The model under review builds one solid part; all positions refer to its coordinate system, in mm. A direction names the side the tool comes from. Round coordinates to 2 decimals unless told otherwise and drop trailing zeros. Order: outer loops, then holes, each group sorted by start corner. A loop starts at its lowest first (then second) coordinate and runs counter-clockwise, first axis right, second up. Notation, with made-up numbers: M 62,50 L 87,50 A13 ccw 87,67 Z; hole C -23.5,-26 d11. An arc over 180 degrees is marked long. Answer as a JSON object with one key per item and string values. Group by question number.
1) Consider section A-A, the plane y = 30. Write out the cut boundary in (x, z).
2) Consider section B-B, the plane x = -20. Write out the cut boundary in (y, z).
3) For faces 1 (the flat face through (8, 12, -24)), 2 (the flat face through (7.5, 32, 0)), 3 (the flat face through (0, 32, 12.5)), 4 (the flat face through (0, 5, 0)), list the 3-axis set-ups (+Z, -Z, +X, -X, +Y, -Y) from which the entire face can be reached by the end or side of a thin tool; tool diameter is ignored.
4) Insertion check: pin 1 Ø8 at (x, y) = (-5.5, 12.5) entering from -Z; pin 2 Ø12 at (y, z) = (6.5, 3.5) entering from +X; pin 3 Ø1 at (y, z) = (20, -19) entering from +X. Each pin has a flat end and moves straight along its axis. Give the tip position at first contact, or say it passes through.
5) To check wall thickness, follow line 1 (Y direction, x = 2, z = -28); line 2 (Z direction, x = 4, y = 25); line 3 (Y direction, x = -11, z = 0). State the ranges of each line that lie inside material, in increasing order.
6) Consider section D-D, the plane z = 20. Write out the cut boundary in (x, y), then the cut area to 3 significant figures.
7) Consider section C-C, the plane y = 7.5. Write out the cut boundary in (x, z).
8) The part is to be moulded in two halves that separate along X. For faces 5 (the cylindrical face through (1.08, 9.86, 21.18)), 6 (the cylindrical face through (7.509, 14.465, 23.846)), 7 (the flat face through (8, 4, -24)), say which applies: +X half, -X half, draft (parallel to the pull), parting line (faces both ways), or undercut.
```python
from build123d import *

# Parameters (mm, degrees)
SKETCH_1_R          = 35
EXTRUDE_1_DEPTH     = 4
SKETCH_2_R          = 25
EXTRUDE_2_DEPTH     = 5
SKETCH_3_R          = 35
EXTRUDE_3_DEPTH     = 3
SKETCH_4_R          = 25
EXTRUDE_4_DEPTH     = 5
SKETCH_5_R          = 35
EXTRUDE_5_DEPTH     = 3
CUT_EXTRUDE_1_REACH = 55.385
SKETCH_6_R          = 1.6
SKETCH_7_R          = 10
CUT_EXTRUDE_2_DEPTH = 5
SKETCH_10_W         = 25
SKETCH_10_H         = 25
SKETCH_10_W_2       = 15
SKETCH_10_H_2       = 15
EXTRUDE_6_DEPTH     = 20
SKETCH_12_R         = 1
CUT_EXTRUDE_5_DEPTH = 20
FILLET_1_R          = 5
SKETCH_13_R         = 1.65
CUT_EXTRUDE_6_DEPTH = 72.282887147
SKETCH_14_R         = 1.65
CUT_EXTRUDE_7_DEPTH = 72.282887147


with BuildPart() as part:
    # 草图1 → 凸台-拉伸1 (new body)
    with BuildSketch(Plane(origin=(0, 0, 0), x_dir=(1, 0, 0), z_dir=(0, 1, 0))):
        with Locations(Location((0, 0, 0), (0, 0, 270))):
            Circle(SKETCH_1_R)
    extrude(amount=EXTRUDE_1_DEPTH)

    # 草图2 → 凸台-拉伸2 (add)
    with BuildSketch(Plane(origin=(0, 4, 0), x_dir=(1, 0, 0), z_dir=(0, 1, 0))):
        with Locations(Location((0, 0, 0), (0, 0, 270))):
            Circle(SKETCH_2_R)
    extrude(amount=EXTRUDE_2_DEPTH)

    # 草图3 → 凸台-拉伸3 (add)
    with BuildSketch(Plane(origin=(0, 9, 0), x_dir=(1, 0, 0), z_dir=(0, 1, 0))):
        with Locations(Location((0, 0, 0), (0, 0, 270))):
            Circle(SKETCH_3_R)
    extrude(amount=EXTRUDE_3_DEPTH)

    # 草图4 → 凸台-拉伸4 (add)
    with BuildSketch(Plane(origin=(0, 12, 0), x_dir=(1, 0, 0), z_dir=(0, 1, 0))):
        with Locations(Location((0, 0, 0), (0, 0, 270))):
            Circle(SKETCH_4_R)
    extrude(amount=EXTRUDE_4_DEPTH)

    # 草图5 → 凸台-拉伸5 (add)
    with BuildSketch(Plane(origin=(0, 17, 0), x_dir=(1, 0, 0), z_dir=(0, 1, 0))):
        with Locations(Location((0, 0, 0), (0, 0, 270))):
            Circle(SKETCH_5_R)
    extrude(amount=EXTRUDE_5_DEPTH)

    # 草图6 → 切除-拉伸1 (cut, up to next)
    with BuildSketch(Plane.XZ, mode=Mode.PRIVATE) as cut_extrude_1_sk1:
        with Locations(Location((-20, 0, 0), (0, 0, 270))):
            Circle(SKETCH_6_R)
    cut_extrude_1_tool1 = extrude(cut_extrude_1_sk1.sketch, amount=-CUT_EXTRUDE_1_REACH, mode=Mode.PRIVATE) & part.part
    # 草图6 → 切除-拉伸1 (cut, up to next)
    with BuildSketch(Plane.XZ, mode=Mode.PRIVATE) as cut_extrude_1_sk2:
        with Locations(Location((0, 20, 0), (0, 0, 270))):
            Circle(SKETCH_6_R)
    cut_extrude_1_tool2 = extrude(cut_extrude_1_sk2.sketch, amount=-CUT_EXTRUDE_1_REACH, mode=Mode.PRIVATE) & part.part
    # 草图6 → 切除-拉伸1 (cut, up to next)
    with BuildSketch(Plane.XZ, mode=Mode.PRIVATE) as cut_extrude_1_sk3:
        with Locations(Location((0, -20, 0), (0, 0, 270))):
            Circle(SKETCH_6_R)
    cut_extrude_1_tool3 = extrude(cut_extrude_1_sk3.sketch, amount=-CUT_EXTRUDE_1_REACH, mode=Mode.PRIVATE) & part.part
    # 草图6 → 切除-拉伸1 (cut, up to next)
    with BuildSketch(Plane.XZ, mode=Mode.PRIVATE) as cut_extrude_1_sk4:
        with Locations(Location((20, 0, 0), (0, 0, 270))):
            Circle(SKETCH_6_R)
    cut_extrude_1_tool4 = extrude(cut_extrude_1_sk4.sketch, amount=-CUT_EXTRUDE_1_REACH, mode=Mode.PRIVATE) & part.part
    add(cut_extrude_1_tool1.solids().sort_by_distance((-20, 0, 0))[0], mode=Mode.SUBTRACT)
    add(cut_extrude_1_tool2.solids().sort_by_distance((0, 0, 20))[0], mode=Mode.SUBTRACT)
    add(cut_extrude_1_tool3.solids().sort_by_distance((0, 0, -20))[0], mode=Mode.SUBTRACT)
    add(cut_extrude_1_tool4.solids().sort_by_distance((20, 0, 0))[0], mode=Mode.SUBTRACT)

    # 草图7 → 切除-拉伸2 (cut)
    with BuildSketch(Plane.XZ):
        with Locations(Location((0, 0, 0), (0, 0, 270))):
            Circle(SKETCH_7_R)
    extrude(amount=-CUT_EXTRUDE_2_DEPTH, mode=Mode.SUBTRACT)

    # 草图10 → 凸台-拉伸6 (add)
    with BuildSketch(Plane(origin=(0, 20, 0), x_dir=(1, 0, 0), z_dir=(0, 1, 0))):
        Rectangle(SKETCH_10_W, SKETCH_10_H)
        Rectangle(SKETCH_10_W_2, SKETCH_10_H_2, mode=Mode.SUBTRACT)
    extrude(amount=EXTRUDE_6_DEPTH)

    # 草图12 → 切除-拉伸5 (cut)
    with BuildSketch(Plane(origin=(0, 40, 0), x_dir=(1, 0, 0), z_dir=(0, 1, 0))):
        with Locations((7.5, 7.5)):
            Circle(SKETCH_12_R)
        with Locations((-7.5, 7.5)):
            Circle(SKETCH_12_R)
        with Locations((-7.5, -7.5)):
            Circle(SKETCH_12_R)
        with Locations((7.5, -7.5)):
            Circle(SKETCH_12_R)
    extrude(amount=-CUT_EXTRUDE_5_DEPTH, mode=Mode.SUBTRACT)

    # 圆角1
    fillet_1_edges = [part.edges().sort_by_distance(p)[0] for p in [
        (12.5, 20, 0),
        (0, 20, -12.5),
        (-12.5, 20, 0),
        (0, 20, 12.5),
    ]]
    fillet(fillet_1_edges, radius=FILLET_1_R)

    # 草图13 → 切除-拉伸6 (cut, through all)
    with BuildSketch(Plane(origin=(12.5, 0, 0), x_dir=(0, 0, -1), z_dir=(1, 0, 0))):
        with Locations((0, 30)):
            Circle(SKETCH_13_R)
    extrude(amount=-CUT_EXTRUDE_6_DEPTH, mode=Mode.SUBTRACT)

    # 草图14 → 切除-拉伸7 (cut, through all)
    with BuildSketch(Plane(origin=(0, 0, -12.5), x_dir=(-1, 0, 0), z_dir=(0, 0, -1))):
        with Locations((0, 35)):
            Circle(SKETCH_14_R)
    extrude(amount=-CUT_EXTRUDE_7_DEPTH, mode=Mode.SUBTRACT)


solid = part.part
```
Results list:
{
 "1": {"outline": "M -12.5,-12.5 L 12.5,-12.5 L 12.5,-1.65 L 7.5,-1.65 L 7.5,-6.5 A1 cw long 6.5,-7.5 L -6.5,-7.5 A1 cw long -7.5,-6.5 L -7.5,-1.65 L -12.5,-1.65 Z; M -12.5,1.65 L -7.5,1.65 L -7.5,6.5 A1 cw long -6.5,7.5 L 6.5,7.5 A1 cw long 7.5,6.5 L 7.5,1.65 L 12.5,1.65 L 12.5,12.5 L -12.5,12.5 Z"},
 "2": {"outline": "M 0,-28.72 L 4,-28.72 L 4,-15 L 9,-15 L 9,-28.72 L 12,-28.72 L 12,-15 L 17,-15 L 17,-28.72 L 20,-28.72 L 20,-1.6 L 0,-1.6 Z; M 0,1.6 L 20,1.6 L 20,28.72 L 17,28.72 L 17,15 L 12,15 L 12,28.72 L 9,28.72 L 9,15 L 4,15 L 4,28.72 L 0,28.72 Z"},
 "3": {"face 1": "none", "face 2": "+Y", "face 3": "+Z, +X, -X, +Y", "face 4": "-Y"},
 "4": {"pin 1": "z = -34.97", "pin 2": "x = 35", "pin 3": "x = 29.71"},
 "5": {"line 1": "0 to 4, 9 to 12, 17 to 20", "line 2": "-12.5 to -7.5, 7.5 to 12.5", "line 3": "0 to 28.35, 31.65 to 40"},
 "6": {"outline": "M -28.72,0 L -1.6,0 L -1.6,20 L -28.72,20 L -28.72,17 L -15,17 L -15,12 L -28.72,12 L -28.72,9 L -15,9 L -15,4 L -28.72,4 Z; M 1.6,0 L 28.72,0 L 28.72,4 L 15,4 L 15,9 L 28.72,9 L 28.72,12 L 15,12 L 15,17 L 28.72,17 L 28.72,20 L 1.6,20 Z", "area": "810 mm^2"},
 "7": {"outline": "C 0,0 d50; hole C -20,0 d3.2; hole C 0,-20 d3.2; hole C 0,20 d3.2; hole C 20,0 d3.2"},
 "8": {"face 5": "undercut", "face 6": "parting line", "face 7": "draft"}
}
